Input: dimensioned drawing with shaded views. Units: mm. Origin: part minimum x, y, z. A direction names the side the tool comes from. Round coordinates to 2 decimals unless told otherwise and drop trailing zeros. Order: outer loops, then holes, each group sorted by start corner. A loop starts at its lowest first (then second) coordinate and runs counter-clockwise, first axis right, second up. Notation, with made-up numbers: M 57.5,34 L 91.5,34 A23 ccw 91.5,69 Z; hole C 19,4 d7. An arc over 180 degrees is marked long. Put each result on its own line as item: value. Start each with the question number.
1) First-contact query: P1, Ø3, axis at x = 21, z = 8, coming from the -Y side; P2, Ø1, axis at x = 33, z = 13, coming from the +Y side; P3, Ø6, axis at y = 13.5, z = 2, coming from the -X side; P4, Ø1, axis at x = 9, y = 11.5, coming from the -Z side. Flat tips, straight axial feed; report the tip coordinate or a pass-through.
2) Section A-A, the plane z = 7.5. Return loops of the section in (x, y), then the cut area to 3 significant figures.
3) Access query for the marked faces 1 and 2. Directions: +Z, -Z, +X, -X, +Y, -Y. A direction counts if a zero-diameter tool reaches every point of the face in a straight line with its end or side. Return the directions, or none.
4) Section C-C, the plane x = 9.5. Return loops of the section in (y, z).
5) Section D-D, the plane x = 24. Return loops of the section in (y, z), then the cut area to 3 significant figures.
6) Material intervals for probe 1 along Y at (x, z) = (32, 7.25); probe 2 along X at (y, z) = (6.5, 0.75); probe 3 along Z at (x, y) = (28.5, 13.5), sorted ascending. Write a range as [from, to].
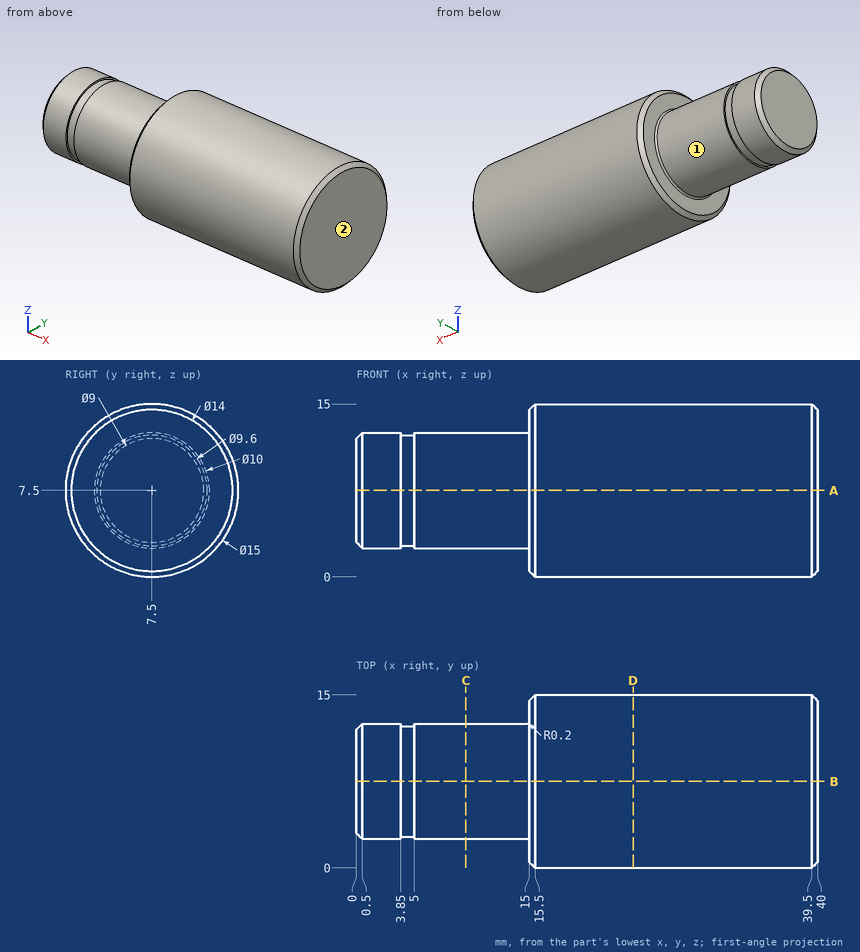
Result sheet:
1. P1: stops at y = 0
1. P2: stops at y = 13.09
1. P3: stops at x = 14.99
1. P4: stops at z = 3.93
2. outline: M 0,3 L 0.5,2.5 L 3.85,2.5 L 3.85,2.7 L 5,2.7 L 5,2.5 L 14.8,2.5 A0.2 cw 15,2.3 L 15,0.5 L 15.5,0 L 39.5,0 L 40,0.5 L 40,14.5 L 39.5,15 L 15.5,15 L 15,14.5 L 15,12.7 A0.2 cw 14.8,12.5 L 5,12.5 L 5,12.3 L 3.85,12.3 L 3.85,12.5 L 0.5,12.5 L 0,12 Z
2. area: 524 mm2
3. face 1: -X
3. face 2: +Z, -Z, +X, +Y, -Y
4. outline: C 7.5,7.5 d10
5. outline: C 7.5,7.5 d15
5. area: 177 mm2
6. probe 1: y = [0, 15]
6. probe 2: x = [15, 40]
6. probe 3: z = [3, 12]
